Here's how the part is built. I have some questions about the finished solid (model axes, mm). Face numbers are marked on the shaded views. A direction names the side the tool comes from. Round coordinates to 2 decimals unless told otherwise and drop trailing zeros. Order: outer loops, then holes, each group sorted by start corner. A loop starts at its lowest first (then second) coordinate and runs counter-clockwise, first axis right, second up. Notation, with made-up numbers: M 61,10.5 L 77,10.5 A24 ccw 77,23.5 Z; hole C 17,-32 d11. An arc over 180 degrees is marked long. Write item = value, one per line. Start each with the question number.
Item 1: I'm going to push a flat-ended pin straight in: P1, Ø1, axis at x = 516.5, z = -278.5, coming from the +Y side. Where does the tip first touch, or does it pass through?
Item 2: I want a section at B-B, the plane y = -146.5. List the corners of the cut face in (x, z) for me, plus the area to 3 significant figures.
Item 3: I want a section at A-A, the plane x = 448.5. List the corners of the cut face in (y, z) for me.
Item 4: We'd pull the mould along Z, two halves only. Please class the marked faces 1, 2 and 3: pulls with the +Z half, pulls with the -Z half, needs draft (parallel to the pull), parting line crosses it, or undercut.
Item 5: Please list where these lines run through material, in increasing order: L1, parallel to X at y = -160.5, z = -90.5; L2, parallel to Y at x = -203.5, z = -100; L3, parallel to X at y = -348.5, z = -240.
Item 6: I want a section at C-C, the plane z = -154. List the corners of the cut face in (x, y) for me.
Item 7: For the marked faces 4 and 5, which set-ups out of +Z, -Z, +X, -X, +Y, -Y let a thin tool reach every point of the face, with its end or its side?
```python
from build123d import *

# Parameters (mm, degrees)
BOSS_EXTRUDE1_DEPTH = 750
SKETCH1_3_W         = 1100
SKETCH1_3_H         = 600
CUT_EXTRUDE1_DEPTH  = 228.6
FILLET1_R           = 50.000000076


with BuildPart() as part:
    # Sketch1 → Boss-Extrude1 (new body)
    with BuildSketch(Plane(origin=(0, 0, 0), x_dir=(1, 0, 0), z_dir=(0, 1, 0))):
        with BuildLine():
            Line((-730, 350), (730, 350))
            ThreePointArc((730, 350), (814.852813742, 314.852813742), (850, 230))
            Line((850, 230), (850, -230))
            ThreePointArc((850, -230), (814.852813742, -314.852813742), (730, -350))
            Line((730, -350), (-730, -350))
            ThreePointArc((-730, -350), (-814.852813742, -314.852813742), (-850, -230))
            Line((-850, -230), (-850, 230))
            ThreePointArc((-850, 230), (-814.852813742, 314.852813742), (-730, 350))
        make_face()
    extrude(amount=-BOSS_EXTRUDE1_DEPTH)

    # Sketch1_3 → Cut-Extrude1 (cut)
    with BuildSketch(Plane(origin=(0, 0, 0), x_dir=(1, 0, 0), z_dir=(0, 1, 0))):
        Rectangle(SKETCH1_3_W, SKETCH1_3_H)
    extrude(amount=-CUT_EXTRUDE1_DEPTH, mode=Mode.SUBTRACT)

    # Fillet1
    fillet1_edges = [part.edges().sort_by_distance(p)[0] for p in [
        (550, -114.3, -300),
        (550, -114.3, 300),
        (-550, -114.3, 300),
        (-550, -114.3, -300),
    ]]
    fillet(fillet1_edges, radius=FILLET1_R)


solid = part.part
```
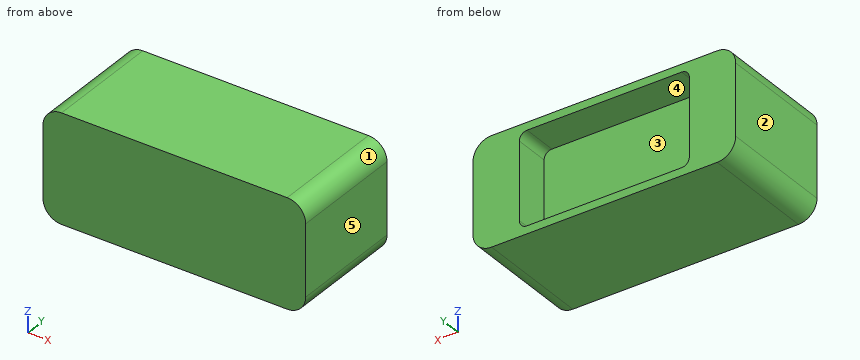
Filled in:
q1.P1 = -228.6
q2.outline = M -850,-230 A120 ccw -730,-350 L 730,-350 A120 ccw 850,-230 L 850,230 A120 ccw 730,350 L -730,350 A120 ccw -850,230 Z; hole M -550,-250 A50 ccw -500,-300 L 500,-300 A50 ccw 550,-250 L 550,250 A50 ccw 500,300 L -500,300 A50 ccw -550,250 Z
q2.area = 520,000 mm^2
q3.outline = M -750,-350 L 0,-350 L 0,-300 L -228.6,-300 L -228.6,300 L 0,300 L 0,350 L -750,350 Z
q4.face_1 = pulls with the +Z half
q4.face_2 = needs draft
q4.face_3 = undercut
q5.L1 = -850 to -550, 550 to 850
q5.L2 = -750 to -228.6
q5.L3 = -849.58 to 849.58
q6.outline = M -850,-750 L 850,-750 L 850,0 L 550,0 L 550,-228.6 L -550,-228.6 L -550,0 L -850,0 Z
q7.face_4 = +Y
q7.face_5 = +Z, -Z, +X, +Y, -Y
